from build123d import *

# Parameters (mm, degrees)
SKETCH1_R           = 30
BOSS_EXTRUDE1_DEPTH = 5
SKETCH2_R           = 30
SKETCH2_R_2         = 22.5
SKETCH2_R_3         = 2.1
SKETCH2_R_4         = 1.5
CUT_EXTRUDE1_DEPTH  = 10
SKETCH3_R           = 14
BOSS_EXTRUDE2_DEPTH = 15
SKETCH4_R           = 2
CUT_EXTRUDE2_DEPTH  = 6
SKETCH5_R           = 7
CUT_EXTRUDE3_DEPTH  = 38.583240946


with BuildPart() as part:
    # Sketch1 → Boss-Extrude1 (new body)
    with BuildSketch(Plane(origin=(0, 0, 0), x_dir=(1, 0, 0), z_dir=(0, 1, 0))):
        with Locations(Location((0, 0, 0), (0, 0, 270))):
            Circle(SKETCH1_R)
    extrude(amount=BOSS_EXTRUDE1_DEPTH)

    # Sketch2 → Cut-Extrude1 (cut)
    # profile 1 of 8: a face of its own
    with BuildSketch(Plane(origin=(0, 0, 0), x_dir=(-1, 0, 0), z_dir=(0, -1, 0))):
        Circle(SKETCH2_R)
        with Locations(Location((0, 0, 0), (0, 0, 90))):
            Circle(SKETCH2_R_2, mode=Mode.SUBTRACT)
    # profile 2 of 8: a face of its own
    with BuildSketch(Plane(origin=(0, 0, 0), x_dir=(-1, 0, 0), z_dir=(0, -1, 0))):
        with Locations(Location((12.019973653, 14.714626511, 0), (0, 0, 90))):
            Circle(SKETCH2_R_3)
    # profile 3 of 8: a face of its own
    with BuildSketch(Plane(origin=(0, 0, 0), x_dir=(-1, 0, 0), z_dir=(0, -1, 0))):
        with Locations(Location((-6.733253539, 17.766915792, 0), (0, 0, 90))):
            Circle(SKETCH2_R_3)
    # profile 4 of 8: a face of its own
    with BuildSketch(Plane(origin=(0, 0, 0), x_dir=(-1, 0, 0), z_dir=(0, -1, 0))):
        with Locations(Location((-18.753227193, 3.052289281, 0), (0, 0, 90))):
            Circle(SKETCH2_R_3)
    # profile 5 of 8: a face of its own
    with BuildSketch(Plane(origin=(0, 0, 0), x_dir=(-1, 0, 0), z_dir=(0, -1, 0))):
        with Locations(Location((-12.019973653, -14.714626511, 0), (0, 0, 90))):
            Circle(SKETCH2_R_3)
    # profile 6 of 8: a face of its own
    with BuildSketch(Plane(origin=(0, 0, 0), x_dir=(-1, 0, 0), z_dir=(0, -1, 0))):
        with Locations(Location((-3.052289281, -18.753227193, 0), (0, 0, 90))):
            Circle(SKETCH2_R_4)
    # profile 7 of 8: a face of its own
    with BuildSketch(Plane(origin=(0, 0, 0), x_dir=(-1, 0, 0), z_dir=(0, -1, 0))):
        with Locations(Location((6.733253539, -17.766915792, 0), (0, 0, 90))):
            Circle(SKETCH2_R_3)
    # profile 8 of 8: a face of its own
    with BuildSketch(Plane(origin=(0, 0, 0), x_dir=(-1, 0, 0), z_dir=(0, -1, 0))):
        with Locations(Location((18.753227193, -3.052289281, 0), (0, 0, 90))):
            Circle(SKETCH2_R_3)
    extrude(amount=-CUT_EXTRUDE1_DEPTH, mode=Mode.SUBTRACT)

    # Sketch3 → Boss-Extrude2 (add)
    with BuildSketch(Plane.XZ):
        with Locations(Location((0, 0, 0), (0, 0, 90))):
            Circle(SKETCH3_R)
    extrude(amount=BOSS_EXTRUDE2_DEPTH)

    # Sketch4 → Cut-Extrude2 (cut)
    with BuildSketch(Plane.XZ.offset(15)):
        with Locations(Location((-0.978927697, 9.951969683, 0), (0, 0, 270))):
            Circle(SKETCH4_R)
        with Locations(Location((-9.951969683, -0.978927697, 0), (0, 0, 270))):
            Circle(SKETCH4_R)
        with Locations(Location((0.978927697, -9.951969683, 0), (0, 0, 270))):
            Circle(SKETCH4_R)
        with Locations(Location((9.951969683, 0.978927697, 0), (0, 0, 270))):
            Circle(SKETCH4_R)
    extrude(amount=-CUT_EXTRUDE2_DEPTH, mode=Mode.SUBTRACT)

    # Sketch5 → Cut-Extrude3 (cut, through all)
    with BuildSketch(Plane.XZ.offset(15)):
        with Locations(Location((0, 0, 0), (0, 0, 270))):
            Circle(SKETCH5_R)
    extrude(amount=-CUT_EXTRUDE3_DEPTH, mode=Mode.SUBTRACT)


solid = part.part
Design review of the part built by this model. Coordinates are the model's own, in mm. A direction names the side the tool comes from. Round coordinates to 2 decimals unless told otherwise and drop trailing zeros. Write each loop counter-clockwise with the first axis right and the second up, starting at its lowest first coordinate (ties: lowest second). Pieces come first, ordered by that corner, then holes. Notation, with made-up numbers: (2, 39) - (56, 39) arc R21 ccw to (56, 70) - close; hole circle Ø10 at (-37, 25). An arc over 180 degrees is marked (long way). Return JSON: item names as keys, results as strings. Group by question number.
Item 1: Machinability: for faces 1 (the face through (16.703, 2.465, -2.597)), 2 (the face through (11.935, -12.042, 1.239)), which of the approach directions +Z, -Z, +X, -X, +Y, -Y give a long, thin tool a straight path to every point of the face, cutting with its end or side? Answer none if there is none.
Item 2: Insertion check: P1, Ø3, axis at y = -9.5, z = 14, coming from the -X side; P2, Ø2, axis at x = -15.5, z = -3, coming from the -Y side; P3, Ø1, axis at y = 0, z = -15.5, coming from the -X side. Each pin has a flat end and moves straight along its axis. Give the tip position at first contact, or say it passes through.
Item 3: For probe 1 along Y at (x, z) = (-21, -1); probe 2 along X at (y, z) = (1.75, -15.5); probe 3 along Z at (x, y) = (-19, 0.5), list the stretches that pass through material, from the lowest coordinate up. Write a range as [from, to].
Item 4: We need section D-D on x = -6. Write out the cut boundary in (y, z), and give its area (3 significant figures).
Item 5: We need section C-C on x = 0. Write out the cut boundary in (y, z).
Item 6: We need section A-A on z = 0. Write out the cut boundary in (x, y), and give its area (3 significant figures).
Item 7: The part is to be moulded in two halves that separate along X. For faces 3 (the face through (-16.67, 2.46, 3.33)), 4 (the face through (5.3, 5, -5.3)), 5 (the face through (-8.618, 2.465, -20.784)), say which applies: pulls with the +X half, pulls with the -X half, needs draft (parallel to the pull), parting line crosses it, or undercut.
Item 8: We need section B-B on y = -2.5. Write out the cut boundary in (x, z).
Model answer:
{
 "1": {"face 1": "+Y, -Y", "face 2": "-Y"},
 "2": {"P1": "stops at x = -6.3", "P2": "stops at y = 0", "P3": "stops at x = -16.77"},
 "3": {"probe 1": "y = [0, 5]", "probe 2": "x = [-16.31, -13.97], [-10.07, 16.31]", "probe 3": "z = [-12.05, 0.97], [5.14, 12.05]"},
 "4": {"outline": "(-15, -12.65) - (0, -12.65) - (0, -21.69) - (5, -21.69) - (5, -3.61) - (-15, -3.61) - close; (-15, 3.61) - (5, 3.61) - (5, 15.8) - (0, 15.8) - (0, 12.65) - (-15, 12.65) - close; (0, 19.73) - (5, 19.73) - (5, 21.69) - (0, 21.69) - close", "area": "432 mm²"},
 "5": {"outline": "(-15, -14) - (0, -14) - (0, -22.5) - (5, -22.5) - (5, -7) - (-15, -7) - (-15, -8.21) - (-9, -8.21) - (-9, -11.7) - (-15, -11.7) - close; (-15, 7) - (5, 7) - (5, 22.5) - (0, 22.5) - (0, 14) - (-15, 14) - (-15, 11.7) - (-9, 11.7) - (-9, 8.21) - (-15, 8.21) - close"},
 "6": {"outline": "(-22.5, 0) - (-14, 0) - (-14, -15) - (-11.7, -15) - (-11.7, -9) - (-8.21, -9) - (-8.21, -15) - (-7, -15) - (-7, 5) - (-22.5, 5) - close; (7, -15) - (8.21, -15) - (8.21, -9) - (11.7, -9) - (11.7, -15) - (14, -15) - (14, 0) - (22.5, 0) - (22.5, 5) - (7, 5) - close", "area": "323 mm²"},
 "7": {"face 3": "undercut", "face 4": "needs draft", "face 5": "parting line crosses it"},
 "8": {"outline": "circle Ø28 at (0, 0); hole circle Ø14 at (0, 0)"}
}
